The drawing under review shows one solid part. Ordinate dimensions are in mm from its lowest x, y, z. A direction names the side the tool comes from. Round coordinates to 2 decimals unless told otherwise and drop trailing zeros. Order: outer loops, then holes, each group sorted by start corner. A loop starts at its lowest first (then second) coordinate and runs counter-clockwise, first axis right, second up. Notation, with made-up numbers: (55, -4.5) -> (63, -4.5) arc R23 cw to (63, 13.5) -> close; hole circle Ø1 at (-3, 66). An arc over 180 degrees is marked (long way). Use a Markdown table: item, result. Add a question column.
1) Wall thickness on line 1 along Z through (x, y) = (10.75, 7.5); line 2 along Y through (x, z) = (3.5, 29); line 3 along X through (y, z) = (0.8, 42.5): over which ranges is each line inside the solid? List them lowest first. Write a range as [from, to].
2) Clearance check with flat-ended pins moving along their axes: P1, Ø3, axis at x = 14, z = 30.5, coming from the -Y side; P2, Ø2, axis at y = 4, z = 5.5, coming from the -X side; P3, Ø2, axis at y = 8.5, z = 22.5, coming from the -X side. State where each tip first meets the part, or that it passes through.
3) Consider section D-D (y = 6.5). State the section outline as (x, z) points.
4) Draft analysis for pull direction Z (two halves, no side actions). For the marked faces 1, 2 and 3, state which applies: pulls with the +Z half, pulls with the -Z half, needs draft (parallel to the pull), parting line crosses it, or undercut.
5) Consider section C-C (y = 1.25). State the section outline as (x, z) points, plus the area to 3 significant figures.
6) Machinability: for the marked faces 4 and 5, which of the approach directions +Z, -Z, +X, -X, +Y, -Y give a long, thin tool a straight path to every point of the face, cutting with its end or side? Answer none if there is none.
7) Consider section B-B (x = 1.75). State the section outline as (y, z) points (1 decimal).
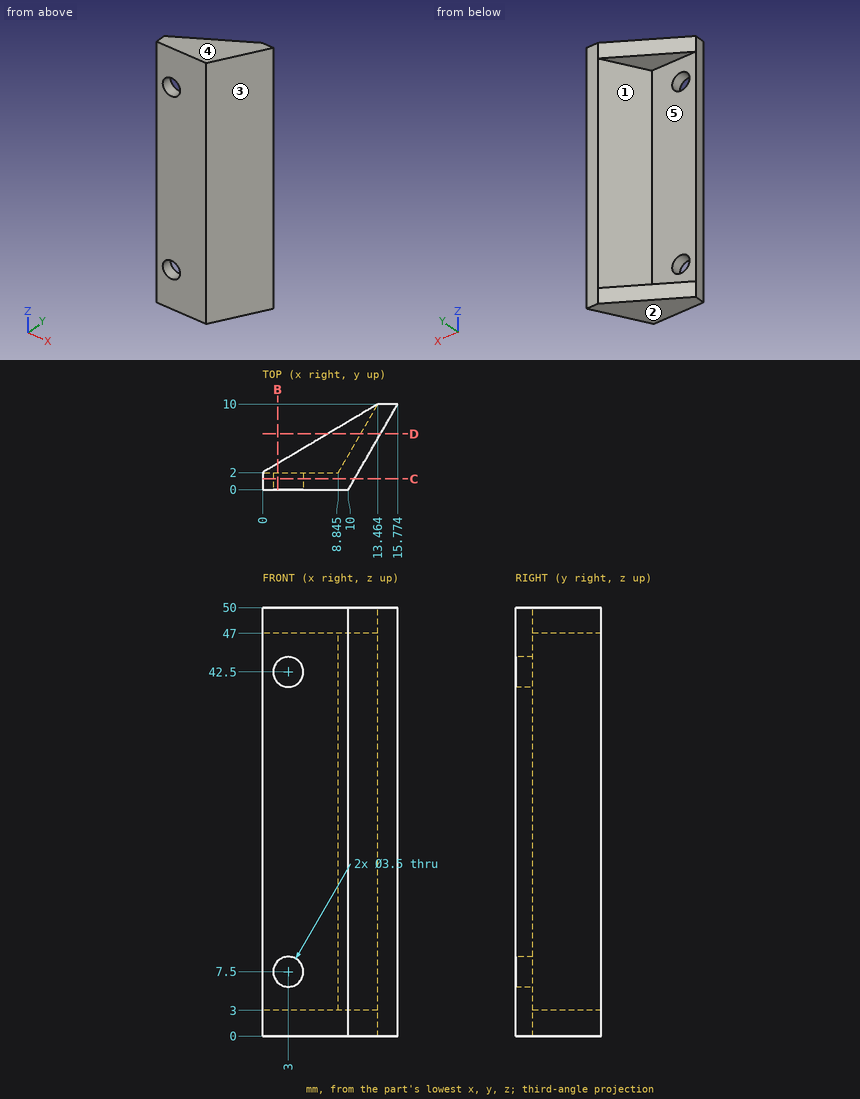
Results list:
| question | item | result |
|---|---|---|
| 1 | line 1 | [0, 3], [47, 50] |
| 1 | line 2 | [0, 2] |
| 1 | line 3 | [0, 1.25], [4.75, 10.46] |
| 2 | P1 | y = 4.33 |
| 2 | P2 | x = 9.42 |
| 2 | P3 | x = 12.02 |
| 3 | outline | (7.57, 0) -> (13.75, 0) -> (13.75, 50) -> (7.57, 50) -> (7.57, 47) -> (11.44, 47) -> (11.44, 3) -> (7.57, 3) -> close |
| 4 | face 1 | undercut |
| 4 | face 2 | pulls with the -Z half |
| 4 | face 3 | needs draft |
| 5 | outline | (0, 0) -> (10.72, 0) -> (10.72, 50) -> (0, 50) -> close; hole circle Ø3.5 at (3, 7.5); hole circle Ø3.5 at (3, 42.5) |
| 5 | area | 517 mm2 |
| 6 | face 4 | +Z, +X, -X, +Y, -Y |
| 6 | face 5 | -X, +Y |
| 7 | outline | (0, 0) -> (3, 0) -> (3, 3) -> (2, 3) -> (2, 6.3) -> (0, 6.3) -> close; (0, 8.7) -> (2, 8.7) -> (2, 41.3) -> (0, 41.3) -> close; (0, 43.7) -> (2, 43.7) -> (2, 47) -> (3, 47) -> (3, 50) -> (0, 50) -> close |
